```python
from build123d import *

# Parameters (mm, degrees)
IZIM1_W                          = 37
IZIM1_H                          = 2
Y_KSEKLIK_EKSTR_ZYON1_DEPTH      = 4.75
Y_KSEKLIK_EKSTR_ZYON2_DEPTH      = 4.75
DELIK1_D                         = 2.95656
DELIK1_DEPTH                     = 2
F_0_15_0_15_DIAMETER_HOLE1_D     = 15
F_0_15_0_15_DIAMETER_HOLE1_DEPTH = 6.75
M7X1_0_TAPPED_HOLE1_D            = 4.5
M7X1_0_TAPPED_HOLE1_DEPTH        = 6.75
M7X1_0_TAPPED_HOLE1_CBORE_D      = 7
M7X1_0_TAPPED_HOLE1_CBORE_DEPTH  = 4


with BuildPart() as part:
    # Çizim1 → Döndür1 (revolve)
    with BuildSketch(Plane(origin=(0, 0, 0), x_dir=(1, 0, 0), z_dir=(0, 1, 0))):
        with Locations((18.5, -1)):
            Rectangle(IZIM1_W, IZIM1_H)
    revolve(axis=Axis((0, 0, 0), (0, 0, 1)))

    # Çizim2 → Yükseklik-Ekstrüzyon1 (add)
    with BuildSketch(Plane.XY.offset(2)):
        with BuildLine():
            Line((-18.2, -22.246481648), (-18.2, 3.246418008))
            ThreePointArc((-18.2, 3.246418008), (-14.7, 12.132116892), (-11.2, 3.246418008))
            Line((-11.2, 3.246418008), (-11.2, -22.246481648))
            ThreePointArc((-11.2, -22.246481648), (-14.7, -31.132180531), (-18.2, -22.246481648))
        make_face()
    extrude(amount=Y_KSEKLIK_EKSTR_ZYON1_DEPTH)

    # Çizim3 → Yükseklik-Ekstrüzyon2 (add)
    with BuildSketch(Plane.XY.offset(2)):
        with BuildLine():
            Line((18.2, 3.246418008), (18.2, -22.246481648))
            ThreePointArc((18.2, -22.246481648), (14.7, -31.132180531), (11.2, -22.246481648))
            Line((11.2, -22.246481648), (11.2, 3.246418008))
            ThreePointArc((11.2, 3.246418008), (14.7, 12.132116892), (18.2, 3.246418008))
        make_face()
    extrude(amount=Y_KSEKLIK_EKSTR_ZYON2_DEPTH)

    # Delik1
    with Locations(Plane.XY.offset(2)):
        with Locations((-30.016940312, -5.292796455), (-26.396454307, 15.24), (-10.424773969, 28.641831082), (10.424773969, 28.641831082), (26.396454307, 15.24), (30.016940312, -5.292796455), (0, -30.48)):
            Hole(DELIK1_D / 2, depth=DELIK1_DEPTH)

    # Ø0.15 (0.15) Diameter Hole1
    with Locations(Plane(origin=(0, 0, 0), x_dir=(-1, 0, 0), z_dir=(0, 0, -1))):
        with Locations((0, 0)):
            Hole(F_0_15_0_15_DIAMETER_HOLE1_D / 2, depth=F_0_15_0_15_DIAMETER_HOLE1_DEPTH)

    # M7x1.0 Tapped Hole1
    with Locations(Plane(origin=(0, 0, 0), x_dir=(-1, 0, 0), z_dir=(0, 0, -1))):
        with Locations((14.7, -26), (-14.7, 6.999957574), (-14.7, -26), (14.7, 6.999957574)):
            CounterBoreHole(M7X1_0_TAPPED_HOLE1_D / 2, M7X1_0_TAPPED_HOLE1_CBORE_D / 2, M7X1_0_TAPPED_HOLE1_CBORE_DEPTH, depth=M7X1_0_TAPPED_HOLE1_DEPTH)


solid = part.part
```
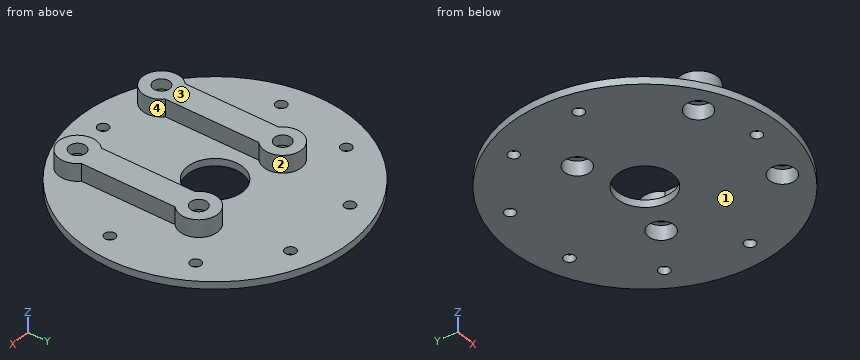
Work out the finished part from the listing and answer in its coordinate system (mm). Face numbers are marked on the shaded views. A direction names the side the tool comes from. Round coordinates to 2 decimals unless told otherwise and drop trailing zeros. Write each loop counter-clockwise with the first axis right and the second up, starting at its lowest first coordinate (ties: lowest second). Pieces come first, ordered by that corner, then holes. Notation, with made-up numbers: (51, -15) -> (100, -15) arc R25 ccw to (100, 3) -> close; hole circle Ø5 at (-11, -30). An arc over 180 degrees is marked (long way). Write each question's results on one line, items separated by ' | '.
Q1. Section D-D, the plane x = -14 is taken. Write down the section's boundary in (y, z).
Data:
outline: (-34.25, 0) -> (-29.43, 0) -> (-29.43, 4) -> (-28.14, 4) -> (-28.14, 6.75) -> (-31.08, 6.75) -> (-31.08, 2) -> (-34.25, 2) -> close; (-23.86, 4) -> (-22.57, 4) -> (-22.57, 0) -> (3.57, 0) -> (3.57, 4) -> (4.86, 4) -> (4.86, 6.75) -> (-23.86, 6.75) -> close; (9.14, 4) -> (10.43, 4) -> (10.43, 0) -> (34.25, 0) -> (34.25, 2) -> (12.08, 2) -> (12.08, 6.75) -> (9.14, 6.75) -> close
Q2. Section A-A, the plane y = 15.24 is taken. Write down the section's boundary in (x, z).
Data:
outline: (-33.72, 0) -> (-27.87, 0) -> (-27.87, 2) -> (-33.72, 2) -> close; (-24.92, 0) -> (24.92, 0) -> (24.92, 2) -> (-24.92, 2) -> close; (27.87, 0) -> (33.72, 0) -> (33.72, 2) -> (27.87, 2) -> close
Q3. Flat-ended cylindrical pins translate along their axes: P1, Ø4, axis at x = -30.02, y = -5.29, coming from the -Z side; P2, Ø4, axis at y = -11.5, z = 5, coming from the -X side; P3, Ø3.5, axis at x = 26.4, y = 15.24, coming from the +Z side; P4, Ø2.5, axis at y = -11.5, z = 5.5, coming from the +X side. Find the tip coordinate at first contact, or state that the pin passes through.
Data:
P1: z = 0 | P2: x = -18.2 | P3: z = 2 | P4: x = 18.2
Q4. Determine the mould class of the marked faces 3 and 4 for opening direction X: released by +X, released by -X, zero draft, split by the parting line, or undercut.
Data:
face 3: zero draft | face 4: undercut
Q5. Section C-C, the plane y = 0 is taken. Write down the section's boundary in (x, z).
Data:
outline: (-37, 0) -> (-7.5, 0) -> (-7.5, 2) -> (-11.2, 2) -> (-11.2, 6.75) -> (-18.2, 6.75) -> (-18.2, 2) -> (-37, 2) -> close; (7.5, 0) -> (37, 0) -> (37, 2) -> (18.2, 2) -> (18.2, 6.75) -> (11.2, 6.75) -> (11.2, 2) -> (7.5, 2) -> close
Q6. Section B-B, the plane x = -5 is taken. Write down the section's boundary in (y, z).
Data:
outline: (-36.66, 0) -> (-5.59, 0) -> (-5.59, 2) -> (-36.66, 2) -> close; (5.59, 0) -> (36.66, 0) -> (36.66, 2) -> (5.59, 2) -> close
Q7. Straight lines are drawn through the part: line 1 along X through (y, z) = (-26.5, 3); line 2 along X through (y, z) = (-27, 1.75); line 3 along X through (y, z) = (0.5, 4.5). For each, find the intervals that lie inside material, in ascending order. Write a range as [from, to].
Data:
line 1: [-19.81, -18.16], [-11.24, -9.59], [9.59, 11.24], [18.16, 19.81] | line 2: [-25.3, -18.05], [-11.35, 11.35], [18.05, 25.3] | line 3: [-18.2, -11.2], [11.2, 18.2]
Q8. Which of the six approach directions +Z, -Z, +X, -X, +Y, -Y give full straight-line access (tool end or side, diameter ignored) to the marked faces 1 and 2?
Data:
face 1: -Z, +X, -X, +Y, -Y | face 2: +Z
